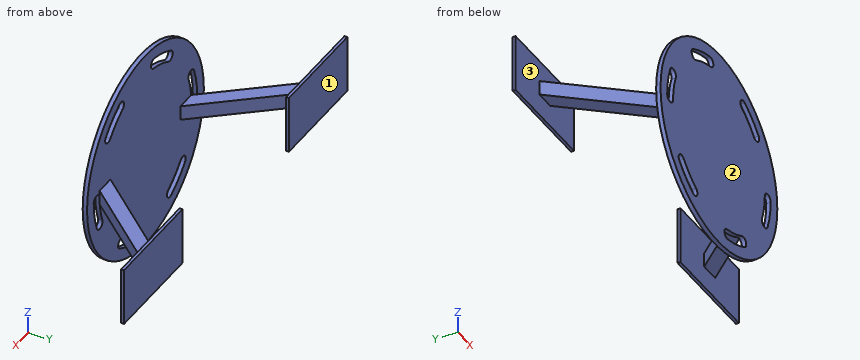
Autodesk Inventor part; units mm, degrees
ref_plane "YZ Plane" through (0, 0, 0) normal (1, 0, 0) x (0, 1, 0)
ref_plane "XZ Plane" through (0, 0, 0) normal (0, 1, 0) x (-1, 0, 0)
ref_plane "XY Plane" through (0, 0, 0) normal (0, 0, 1) x (1, 0, 0)
sketch "Sketch1" plane through (0, 0, 0) normal (0, 1, 0) x (-1, 0, 0)
  circle A0 centre (0, 0) radius 70
  dimension "d0" = 140
extrude "Extrusion1" add sketch "Sketch1" along normal blind 3
sketch "Sketch2" plane through (0, 3, 0) normal (0, 1, 0) x (1, 0, 0)
  circle A0 centre (0, 0) radius 62
  circle A1 centre (0, 0) radius 55
  arc A2 (-55, 0) -> (-62, 0) centre (-58.5, 0) ccw
  arc A3 (-58.2641, -21.1966) -> (-51.6859, -18.8034) centre (-54.975, -20) ccw
  dimension "d3" = 124
  dimension "d4" = 110
  dimension "d7" = 20
extrude "Extrusion2" cut sketch "Sketch2" against normal through all contours A2 A1 A3 A0 picked at (-56.7601, -18.0974)
pattern_circular "Circular Pattern1" count 6 over 360 about axis through (0, 0, 0) along (0, 1, 0) of "Extrusion2"
sketch "Sketch4" plane through (0, 0, 0) normal (0, 0, 1) x (1, 0, 0)
  line L0 (70, 3) -> (-70, 3)
  line L1 (-41.9459, 3) -> (-92.2919, 63)
  line L2 (-92.2919, 63) -> (-105.346, 63)
  line L3 (-105.346, 63) -> (-55, 3)
  point P0 (0, 0)
  point P1 (0, 3)
  dimension "d13" = 50
  dimension "d14" = 60
  dimension "d15" = 55
  dimension "d16" = 10
extrude "Extrusion3" add sketch "Sketch4" along normal mid plane 10
mirror "Mirror1" about plane through (0, 0, 0) normal (1, 0, 0) of "Extrusion3"
sketch "Sketch6" plane through (0, 0, 0) normal (0, 0, 1) x (1, 0, 0)
  line L0 (-63.8189, 65) -> (-133.8189, 65)
  line L1 (-133.8189, 65) -> (-133.8189, 63)
  line L2 (-133.8189, 63) -> (-63.8189, 63)
  line L3 (-63.8189, 63) -> (-63.8189, 65)
  line L4 (-63.8189, 65) -> (-133.8189, 63) construction
  line L5 (-133.8189, 65) -> (-63.8189, 63) construction
  line L6 (-105.346, 63) -> (-92.2919, 63)
  point P0 (0, 0)
  point P1 (-98.8189, 64)
  point P2 (-98.8189, 63)
  point P3 (-98.8189, 63)
  dimension "d22" = 2
  dimension "d23" = 70
  dimension "d24" = 0
extrude "Extrusion4" add sketch "Sketch6" along normal mid plane 40
mirror "Mirror2" about plane through (0, 0, 0) normal (1, 0, 0) of "Extrusion4"
properties part number "Bottom_plate"
Design review of the part built by this model. Coordinates are the model's own, in mm. Face numbers are marked on the shaded views. Coordinates: 2 decimals unless noted, no trailing zeros. Order: outer loops, then holes, each group sorted by start corner. A loop starts at its lowest first (then second) coordinate and runs counter-clockwise, first axis right, second up. Notation, with made-up numbers: M -3,8 L 8,8 A34 cw 8,46 Z; hole C -33.5,28 d9. An arc over 180 degrees is marked long. Answer as a JSON object with one key per item and string values. Group by question number.
1) Wall thickness on L1, parallel to Y at x = 66, z = -18; L2, parallel to Y at x = 30.5, z = 27.5; L3, parallel to Z at x = -101.5, y = 58.5: over which ranges is each line inside the solid? List them lowest first.
2) Add section A-A, the plane z = 15.5. Write out the cut boundary in (x, y).
3) Add section D-D, the plane x = -100. Write out the cut boundary in (y, z), then the cut area to 3 significant figures.
4) Add section C-C, the plane x = 81.5. Write out the cut boundary in (y, z).
5) Add section B-B, the plane y = 44.5. Write out the cut boundary in (x, z).
6) Mouldability with a two-part tool opening along Y and no side actions: class the marked faces 1, 2 and 3 as pulls with the +Y half, pulls with the -Y half, needs draft (parallel to the pull), parting line crosses it, or undercut.
7) For pin 1 (6 mm diameter, centred on x = 12.5, z = 43.5, fed in from +Y); pin 2 (3 mm diameter, centred on x = 31.5, z = 18, fed in from -Y); pin 3 (2 mm diameter, centred on x = -114.5, y = 64, fed in from +Z); pin 4 (1.5 mm diameter, centred on x = 86.5, y = 57.5, fed in from -Z), all flat-tipped, find the tip position at first contact; note any pin that passes through.
Computed values:
{
 "1": {"L1": "y = 0 to 3, 63 to 65", "L2": "y = 0 to 3", "L3": "z = -5 to 5"},
 "2": {"outline": "M -133.82,63 L -63.82,63 L -63.82,65 L -133.82,65 Z; M -68.26,0 L -60.03,0 L -60.03,3 L -68.26,3 Z; M -52.77,0 L 68.26,0 L 68.26,3 L -52.77,3 Z; M 63.82,63 L 133.82,63 L 133.82,65 L 63.82,65 Z"},
 "3": {"outline": "M 56.63,-5 L 63,-5 L 63,-20 L 65,-20 L 65,20 L 63,20 L 63,5 L 56.63,5 Z", "area": "144 mm^2"},
 "4": {"outline": "M 34.58,-5 L 50.14,-5 L 50.14,5 L 34.58,5 Z; M 63,-20 L 65,-20 L 65,20 L 63,20 Z"},
 "5": {"outline": "M -89.82,-5 L -76.77,-5 L -76.77,5 L -89.82,5 Z; M 76.77,-5 L 89.82,-5 L 89.82,5 L 76.77,5 Z"},
 "6": {"face 1": "pulls with the +Y half", "face 2": "pulls with the -Y half", "face 3": "undercut"},
 "7": {"pin 1": "stops at y = 3", "pin 2": "stops at y = 0", "pin 3": "stops at z = 20", "pin 4": "passes through"}
}
